Read the model definition and answer for the solid it produces. Units are mm, in the model's axes. Coordinates: 2 decimals unless noted, no trailing zeros. Write each loop counter-clockwise with the first axis right and the second up, starting at its lowest first coordinate (ties: lowest second). Pieces come first, ordered by that corner, then holes.
Item 1: This flat-tipped pin is pushed along its axis until it touches: P1, Ø5, axis at x = 91.44, z = -10.16, coming from the -Y side. Where does it stop, or does it pass through?
Item 2: Determine the mould class of faces 1 (the face through (1, 0, -100)), 2 (the face through (-7.13, 1.93, -11.11)) for opening direction X: released by +X, released by -X, zero draft, split by the parting line, or undercut.
Item 3: Section B-B (x = 10.16) is taken. Give the vertices of the cut face in (y, z) (3 decimals), then the cut area to 3 significant figures.
Item 4: Section A-A (z = -193.04) is taken. Give the vertices of the cut face in (x, y) (3 decimals).
Item 5: Section C-C (z = -10.16) is taken. Give the vertices of the cut face in (x, y) (3 decimals), then the cut area to 3 significant figures.
Item 6: Straight lines are drawn through the part: probe 1 along X at (y, z) = (1.95, -10.16) (3 decimals); probe 2 along Z at (x, y) = (91.5, 0.6); probe 3 along X at (y, z) = (3.65, -136.5). For each, find the intervals that lie inside material, in ascending order.
Item 7: Section D-D (x = 91.44) is taken. Give the vertices of the cut face in (y, z) (3 decimals), then the cut area to 3 significant figures.
Autodesk Inventor part; units mm, degrees
ref_plane "YZ Plane" through (0, 0, 0) normal (1, 0, 0) x (0, 1, 0)
ref_plane "XZ Plane" through (0, 0, 0) normal (0, 1, 0) x (-1, 0, 0)
ref_plane "XY Plane" through (0, 0, 0) normal (0, 0, 1) x (1, 0, 0)
sketch "Sketch1" plane through (0, 0, 0) normal (0, 1, 0) x (-1, 0, 0)
  line L0 (101.6, 0) -> (-101.6, 0)
  line L1 (-101.6, 0) -> (-101.6, -203.2)
  line L2 (-101.6, -203.2) -> (101.6, -203.2)
  line L3 (101.6, -203.2) -> (101.6, 0)
  dimension "d0" = 203.2
  dimension "d1" = 203.2
extrude "Extrusion1" add sketch "Sketch1" along normal blind 3.81
sketch "Sketch2" plane through (0, 3.81, 0) normal (0, 1, 0) x (1, 0, 0)
  circle A0 centre (-91.44, 10.16) radius 10.16
  circle A1 centre (-91.44, 10.16) radius 3.175
  line L0 (-101.6, 203.2) -> (-101.6, 0)
  line L1 (-101.6, 101.6) -> (101.6, 101.6)
  line L2 (101.6, 0) -> (101.6, 203.2)
  line L3 (-101.6, 0) -> (101.6, 0)
  line L4 (0, 0) -> (0, 101.6)
  circle A2 centre (91.44, 10.16) radius 10.16
  circle A3 centre (91.44, 10.16) radius 3.175
  circle A4 centre (-91.44, 193.04) radius 10.16
  circle A5 centre (-91.44, 193.04) radius 3.175
  circle A6 centre (91.44, 193.04) radius 10.16
  circle A7 centre (91.44, 193.04) radius 3.175
  point P0 (0, 0)
  dimension "d4" = 20.32
  dimension "d5" = 6.35
extrude "Extrusion2" cut sketch "Sketch2" against normal blind 3.81 contours A1 | A3 | A5 | A7
sketch "Sketch3" plane through (0, 3.81, 0) normal (0, 1, 0) x (1, 0, 0)
  line L0 (101.6, 0) -> (101.6, 203.2)
  line L1 (101.6, 101.6) -> (-101.6, 101.6)
  line L2 (-101.6, 203.2) -> (-101.6, 0)
  circle A0 centre (-91.44, 111.76) radius 10.16
  circle A1 centre (-91.44, 111.76) radius 3.175
  circle A2 centre (91.44, 111.76) radius 10.16
  circle A3 centre (91.44, 111.76) radius 3.175
  point P0 (-100.0125, 103.1875)
  dimension "d8" = 20.32
  dimension "d9" = 6.35
  dimension "d10" = 20.32
  dimension "d11" = 6.35
extrude "Extrusion3" cut sketch "Sketch3" against normal blind 3.81 contours A1 | A3
sketch "Sketch4" plane through (0, 3.81, 0) normal (0, 1, 0) x (1, 0, 0)
  circle A0 centre (-48.895, 113.03) radius 1.5
  circle A1 centre (-48.895, 113.03) radius 1.5
  circle A2 centre (-8.255, 113.03) radius 1.5
  circle A3 centre (-8.255, 113.03) radius 1.5
  line L0 (-3.175, 107.95) -> (-13.335, 107.95)
  line L1 (-53.975, 130.175) -> (-53.975, 107.95)
  line L2 (-3.175, 107.95) -> (-53.975, 107.95)
  line L3 (-53.975, 107.95) -> (-53.975, 132.715)
  line L4 (-53.975, 132.715) -> (-3.175, 132.715)
  line L5 (-3.175, 132.715) -> (-3.175, 107.95)
  line L6 (-101.6, 203.2) -> (-101.6, 0)
  line L7 (101.6, 0) -> (101.6, 203.2)
  line L8 (-101.6, 0) -> (101.6, 0)
  line L9 (101.6, 0) -> (101.6, 107.95)
  line L10 (101.6, 107.95) -> (-101.6, 107.95)
  line L11 (-101.6, 107.95) -> (-101.6, 0)
  line L12 (-53.975, 120.3325) -> (-3.175, 120.3325)
  circle A4 centre (-48.895, 127.635) radius 1.5
  circle A5 centre (-48.895, 127.635) radius 1.5
  circle A6 centre (-8.255, 127.635) radius 1.5
  circle A7 centre (-8.255, 127.635) radius 1.5
  line L13 (-48.895, 107.95) -> (-48.895, 113.03)
  line L14 (-8.255, 107.95) -> (-8.255, 113.03)
  line L15 (-8.255, 132.715) -> (-8.255, 127.635)
  line L16 (-48.895, 132.715) -> (-48.895, 127.635)
  dimension "d14" = 107.95
extrude "Extrusion4" cut sketch "Sketch4" against normal blind 3.81 contours A0 | A2 | A6 | A4
sketch "Sketch5" plane through (0, 3.81, 0) normal (0, 1, 0) x (1, 0, 0)
  circle A0 centre (10.16, 10.16) radius 10.16
  circle A1 centre (10.16, 10.16) radius 3.175
  line L0 (-101.6, 0) -> (101.6, 0)
  line L1 (101.6, 203.2) -> (-101.6, 203.2)
  line L2 (0, 203.2) -> (0, 150.8125)
  circle A2 centre (-10.16, 10.16) radius 10.16
  circle A3 centre (-10.16, 10.16) radius 3.175
  dimension "d17" = 20.32
  dimension "d18" = 6.35
extrude "Extrusion5" cut sketch "Sketch5" against normal blind 3.81 contours A1 | A3
sketch "Sketch6" plane through (0, 3.81, 0) normal (0, 1, 0) x (1, 0, 0)
  line L0 (-44.1448, 101.6) -> (0, 101.6)
  line L1 (0, 101.6) -> (0, 136.525)
  line L2 (0, 136.525) -> (-44.1448, 136.525)
  line L3 (-44.1448, 136.525) -> (-44.1448, 101.6)
  circle A0 centre (-40.1448, 132.5875) radius 1.5
  circle A1 centre (-40.1448, 132.5875) radius 1.5
  circle A2 centre (-40.1448, 105.5375) radius 1.5
  circle A3 centre (-40.1448, 105.5375) radius 1.5
  circle A4 centre (-4, 105.5375) radius 1.5
  circle A5 centre (-4, 105.5375) radius 1.5
  circle A6 centre (-4, 132.5875) radius 1.5
  circle A7 centre (-4, 132.5875) radius 1.5
  line L4 (-101.6, 203.2) -> (-101.6, 0)
  line L5 (-101.6, 101.6) -> (101.6, 101.6)
  line L6 (101.6, 0) -> (101.6, 203.2)
extrude "Extrusion6" cut sketch "Sketch6" against normal blind 3.81 contours A0 | A2 | A4 | A6
sketch "Sketch7" plane through (0, 3.81, 0) normal (0, 1, 0) x (1, 0, 0)
  circle A0 centre (2.54, 15.24) radius 1.5875
  circle A1 centre (2.54, 15.24) radius 1.5875
  circle A2 centre (50.8, 13.97) radius 1.5875
  circle A3 centre (45.72, 66.04) radius 1.5875
  circle A4 centre (17.78, 66.04) radius 1.5875
  circle A5 centre (50.8, 13.97) radius 1.5875
  line L0 (50.8, 13.97) -> (50.8, 0)
  line L1 (0, 0) -> (53.34, 0)
  line L2 (50.8, 0) -> (53.34, 0)
  line L3 (53.34, 0) -> (53.34, 66.04)
  line L4 (53.34, 66.04) -> (53.34, 68.58)
  line L5 (53.34, 68.58) -> (0, 68.58)
  line L6 (0, 68.58) -> (0, 0)
  line L7 (0, 0) -> (53.34, 0)
  line L8 (2.54, 15.24) -> (0, 15.24)
  line L9 (0, 66.04) -> (0, 0)
  circle A6 centre (17.78, 66.04) radius 1.5875
  line L10 (17.78, 66.04) -> (17.78, 68.58)
  line L11 (45.72, 66.04) -> (45.72, 68.58)
  line L12 (23.5657, 188.7512) -> (23.5657, 202.7212)
  circle A7 centre (23.5657, 188.7512) radius 1.5875
  line L13 (23.5657, 202.7212) -> (21.0257, 202.7212)
  line L14 (74.3657, 202.7212) -> (21.0257, 202.7212)
  line L15 (74.3657, 202.7212) -> (21.0257, 202.7212)
  line L16 (74.3657, 136.6812) -> (74.3657, 202.7212)
  line L17 (74.3657, 134.1412) -> (74.3657, 202.7212)
  line L18 (21.0257, 202.7212) -> (21.0257, 136.6812)
  circle A8 centre (56.5857, 136.6812) radius 1.5875
  circle A9 centre (56.5857, 136.6812) radius 1.5875
  line L19 (56.5857, 136.6812) -> (56.5857, 134.1412)
  line L20 (21.0257, 134.1412) -> (74.3657, 134.1412)
  line L21 (28.6457, 136.6812) -> (28.6457, 134.1412)
  circle A10 centre (28.6457, 136.6812) radius 1.5875
  line L22 (21.0257, 136.6812) -> (21.0257, 134.1412)
  circle A11 centre (71.8257, 187.4812) radius 1.5875
  circle A12 centre (71.8257, 187.4812) radius 1.5875
  line L23 (71.8257, 187.4812) -> (74.3657, 187.4812)
  circle A13 centre (23.5657, 188.7512) radius 1.5875
  point P0 (71.8257, 187.4812)
extrude "Extrusion7" cut sketch "Sketch7" against normal blind 3.81 contours A10 | A8 | A11 | A7
properties part number "grounplate" material "Wood (Birch)"
Established:
1. P1: passes through
2. face 1: zero draft
2. face 2: undercut
3. outline: (0, -203.2) - (3.81, -203.2) - (3.81, -13.335) - (0, -13.335) - close; (0, -6.985) - (3.81, -6.985) - (3.81, 0) - (0, 0) - close
3. area: 750 mm2
4. outline: (-101.6, 0) - (-94.615, 0) - (-94.615, 3.81) - (-101.6, 3.81) - close; (-88.265, 0) - (88.265, 0) - (88.265, 3.81) - (-88.265, 3.81) - close; (94.615, 0) - (101.6, 0) - (101.6, 3.81) - (94.615, 3.81) - close
5. outline: (-101.6, 0) - (-94.615, 0) - (-94.615, 3.81) - (-101.6, 3.81) - close; (-88.265, 0) - (-13.335, 0) - (-13.335, 3.81) - (-88.265, 3.81) - close; (-6.985, 0) - (6.985, 0) - (6.985, 3.81) - (-6.985, 3.81) - close; (13.335, 0) - (88.265, 0) - (88.265, 3.81) - (13.335, 3.81) - close; (94.615, 0) - (101.6, 0) - (101.6, 3.81) - (94.615, 3.81) - close
5. area: 677 mm2
6. probe 1: x = -101.6 to -94.615, -88.265 to -13.335, -6.985 to 6.985, 13.335 to 88.265, 94.615 to 101.6
6. probe 2: z = -203.2 to -196.21, -189.87 to -114.93, -108.59 to -13.33, -6.99 to 0
6. probe 3: x = -101.6 to 27.07, 30.22 to 55.01, 58.16 to 101.6
7. outline: (0, -203.2) - (3.81, -203.2) - (3.81, -196.215) - (0, -196.215) - close; (0, -189.865) - (3.81, -189.865) - (3.81, -114.935) - (0, -114.935) - close; (0, -108.585) - (3.81, -108.585) - (3.81, -13.335) - (0, -13.335) - close; (0, -6.985) - (3.81, -6.985) - (3.81, 0) - (0, 0) - close
7. area: 702 mm2
